Input: part model. Units: mm. Frame: model coordinates. A direction names the side the tool comes from. Coordinates: 2 decimals unless noted, no trailing zeros. Loops run counter-clockwise (first coordinate to the right, second up) from the corner with the lowest first, then second, coordinate; pieces in that order, holes last. Notation, with made-up numbers: (89.25, 22) - (119.25, 22) arc R11 cw to (119.25, 27) - close; hole circle Ø1 at (-2, -21.75). An arc over 180 degrees is marked (long way). Use a Markdown table: item, result. Add a question column.
1. Section query D-D on x = 38. Return the cut outline in (y, z) (3 decimals).
2. Section query B-B on z = 9.5. Return the cut outline in (x, y) (3 decimals).
3. Section query A-A on x = 8.5. Return the cut outline in (y, z).
4. Ray query, L1, parallel to Y at x = 20.5, z = 12.5 (3 decimals); L2, parallel to Y at x = 4, z = 16; L3, parallel to Y at x = 6.5, z = 21. Return the intervals inside material, ascending. Write a range as [from, to].
5. Contact query for flat-ended pins moving along their axis: P1, Ø1, axis at y = 16, z = 8.5, coming from the +X side; P2, Ø7.5, axis at y = 19.5, z = 22.5, coming from the +X side; P3, Ø2, axis at x = 33, z = 3.5, coming from the +Y side (3 decimals). Output: stop coordinate, or through.
6. Draft query along Y for faces 1 (the face through (43.942, 7, 16)), 2 (the face through (10, 25.4, 16)), 3 (the face through (23, 0, 16)), 4 (the face through (12.7, 12.9, 15.7)). Return one class per face: released by +Y, released by -Y, zero draft, split by the parting line, or undercut.
7. Access query for faces 5 (the face through (28, 10, 31.75)), 6 (the face through (36, 15.875, 16)). Directions: +Z, -Z, +X, -X, +Y, -Y. A direction counts if a zero-diameter tool reaches every point of the face in a straight line with its end or side. Return the directions, or none.
```python
from build123d import *

# Parameters (mm, degrees)
BOSS_EXTRUDE1_DEPTH      = 31.75
X_0_397_DIAMETER_HOLE1_D = 10.795
CHAMFER1_SIZE            = 1.27
CHAMFER2_SIZE            = 0.254
FILLET1_R                = 0.254


with BuildPart() as part:
    # Sketch1 → Boss-Extrude1 (new body)
    with BuildSketch(Plane.XY):
        with BuildLine():
            Line((2.54, 0), (43.942, 0))
            Line((43.942, 0), (43.942, 15.875))
            Line((43.942, 15.875), (17.399, 15.875))
            Line((17.399, 15.875), (17.399, 25.4))
            Line((17.399, 25.4), (2.54, 25.4))
            Line((2.54, 25.4), (2.54, 25.143407893))
            ThreePointArc((2.54, 25.143407893), (12.7, 12.7), (2.54, 0.256592107))
            Line((2.54, 0.256592107), (2.54, 0))
        make_face()
    extrude(amount=BOSS_EXTRUDE1_DEPTH)

    # X (0.397) Diameter Hole1 (through all)
    with Locations(Plane(origin=(0, 15.875, 0), x_dir=(1, 0, 0), z_dir=(0, 1, 0))):
        with Locations((29.718, -15.875)):
            Hole(X_0_397_DIAMETER_HOLE1_D / 2)

    # Chamfer1
    chamfer1_edges = [part.edges().sort_by_distance(p)[0] for p in [
        (43.942, 15.875, 15.875),
    ]]
    chamfer(chamfer1_edges, length=CHAMFER1_SIZE)

    # Chamfer2
    chamfer2_edges = [part.edges().sort_by_distance(p)[0] for p in [
        (35.1155, 15.875, 15.875),
    ]]
    chamfer(chamfer2_edges, length=CHAMFER2_SIZE)

    # Fillet1
    fillet1_edges = [part.edges().sort_by_distance(p)[0] for p in [
        (17.399, 15.875, 15.875),
    ]]
    fillet(fillet1_edges, radius=FILLET1_R)


solid = part.part
```
Resolved:
| question | item | result |
|---|---|---|
| 1 | outline | (0, 0) - (15.875, 0) - (15.875, 31.75) - (0, 31.75) - close |
| 2 | outline | (2.54, 0) - (43.942, 0) - (43.942, 14.605) - (42.672, 15.875) - (17.653, 15.875) arc R0.254 cw to (17.399, 16.129) - (17.399, 25.4) - (2.54, 25.4) - (2.54, 25.143) arc R12.7 cw to (2.54, 0.257) - close |
| 3 | outline | (0, 0) - (3.26, 0) - (3.26, 31.75) - (0, 31.75) - close; (22.14, 0) - (25.4, 0) - (25.4, 31.75) - (22.14, 31.75) - close |
| 4 | L1 | [0, 15.875] |
| 4 | L2 | [0, 0.65], [24.75, 25.4] |
| 4 | L3 | [0, 1.79], [23.61, 25.4] |
| 5 | P1 | x = 43.05 |
| 5 | P2 | x = 42.8 |
| 5 | P3 | y = 15.875 |
| 6 | face 1 | zero draft |
| 6 | face 2 | released by +Y |
| 6 | face 3 | released by -Y |
| 6 | face 4 | undercut |
| 7 | face 5 | +Z, +X, -X, +Y, -Y |
| 7 | face 6 | +Z, -Z, +X, +Y |
